Source: CAD feature listing. Evaluate the final solid. Frame: model axes, mm. A direction names the side the tool comes from. Round coordinates to 2 decimals unless told otherwise and drop trailing zeros. Order: outer loops, then holes, each group sorted by start corner. A loop starts at its lowest first (then second) coordinate and runs counter-clockwise, first axis right, second up. Notation, with made-up numbers: (84, 81.5) - (113, 81.5) arc R20 cw to (113, 90.5) - close; hole circle Ø7 at (79, 19.5). An arc over 180 degrees is marked (long way). Put each result on its own line as item: value. Start each with the question number.
1) Line query: probe 1 along X at (y, z) = (-3.5, 1.75); probe 2 along Y at (x, z) = (-6.5, -1); probe 3 along Y at (x, z) = (0.75, 2.25). Output: solid intervals per line, ascending. Write a range as [from, to].
2) Mould query, pull axis X, two halves, no side actions, for faces 1 (the face through (-6, -3.25, 2)), 2 (the face through (7, -5, -1)), 3 (the face through (-6.24, 3.826, -3.073)). Classes: +X half, -X half, draft (parallel to the pull), parting line (faces both ways), or undercut.
3) Section C-C on x = 3.25. Output: boundary loops of the cut face in (y, z), then the cut area to 3 significant figures.
4) Access query for faces 4 (the face through (-5, 2, 2)), 5 (the face through (-6.6, -5.75, -1.5)), 6 (the face through (-4, 0, 4.2)), 7 (the face through (-6.6, 3.75, -1.5)), 8 (the face through (0, 5, 1)). Directions: +Z, -Z, +X, -X, +Y, -Y. A direction counts if a zero-diameter tool reaches every point of the face in a straight line with its end or side. Return the directions, or none.
5) Section D-D on y = 3.5. Output: boundary loops of the cut face in (x, z) (3 decimals), then the cut area to 3 significant figures.
6) Section A-A on y = -3. Output: boundary loops of the cut face in (x, z).
7) Contact query for flat-ended pins moving along their axis: P1, Ø1.5, axis at y = 5, z = 3, coming from the +X side; P2, Ø1.2, axis at y = -0.5, z = 1.5, coming from the +X side (3 decimals); P3, Ø2, axis at y = -5.5, z = -0.5, coming from the +X side; P4, Ø0.6, axis at x = 6, y = 5, coming from the +Z side. Output: stop coordinate, or through.
8) Section B-B on z = -1. Output: boundary loops of the cut face in (x, y), then the cut area to 3 significant figures.
```python
from build123d import *
from OCP.BRepFilletAPI import BRepFilletAPI_MakeChamfer

# Parameters (mm, degrees)
ESQUISSE1_W             = 14.5
ESQUISSE1_H             = 14.5
BOSS_EXTRU_1_DEPTH      = 5
ESQUISSE2_W             = 8
ESQUISSE2_H             = 6.5
ENL_V_MAT_EXTRU_1_DEPTH = 12.407234547
CHANFREIN1_SIZE         = 5
CHANFREIN1_SIZE_2       = 1.75
CHANFREIN2_SIZE         = 5
CHANFREIN2_SIZE_2       = 3
ESQUISSE3_W             = 2
ESQUISSE3_H             = 4
ENL_V_MAT_EXTRU_2_DEPTH = 3.5
ESQUISSE6_W             = 10
ESQUISSE6_H             = 3
ENL_V_MAT_EXTRU_3_DEPTH = 4
CHANFREIN3_SIZE         = 4
CHANFREIN3_SIZE2        = 1.5
CONG_1_R                = 2
ESQUISSE7_W             = 1.25
ESQUISSE7_H             = 4
ENL_V_MAT_EXTRU_4_DEPTH = 4
ESQUISSE8_W             = 1.5
ESQUISSE8_H             = 2
BOSS_EXTRU_2_DEPTH      = 4
CHANFREIN4_SIZE         = 0.2
CHANFREIN4_SIZE2        = 1.5
CHANFREIN5_SIZE         = 1.5
CHANFREIN5_SIZE2        = 0.2
CHANFREIN6_SIZE         = 0.5
CHANFREIN6_SIZE2        = 1.5
CHANFREIN7_SIZE         = 1.5
CHANFREIN7_SIZE2        = 0.5
ESQUISSE9_W             = 1
ESQUISSE9_H             = 3
ENL_V_MAT_EXTRU_5_DEPTH = 3.5
ESQUISSE10_W            = 4.75
ESQUISSE10_H            = 1
ENL_V_MAT_EXTRU_6_DEPTH = 12.407234547
ESQUISSE11_W            = 1.5
ESQUISSE11_H            = 0.5
ENL_V_MAT_EXTRU_7_DEPTH = 4.25
CONG_2_START            = -3.497851783
CONG_2_DEPTH            = 7


with BuildPart() as part:
    # Esquisse1 → Boss.-Extru.1 (new body)
    with BuildSketch(Plane.XY):
        Rectangle(ESQUISSE1_W, ESQUISSE1_H)
    extrude(amount=BOSS_EXTRU_1_DEPTH)

    # Esquisse2 → Enlèv. mat.-Extru.1 (cut, through all)
    with BuildSketch(Plane.XY.offset(5)):
        Rectangle(ESQUISSE2_W, ESQUISSE2_H)
    extrude(amount=-ENL_V_MAT_EXTRU_1_DEPTH, mode=Mode.SUBTRACT)

    # Chanfrein1
    # the kernel refuses this chamfer: 5, 1.75 mm, written as the material it takes off along each edge
    with BuildSketch(Plane(origin=(7.25, 20.222980747, 5), x_dir=(0, 0, -1), z_dir=(0, -1, 0)), Plane(origin=(-7.25, -20.222980747, 5), x_dir=(0, 0, -1), z_dir=(0, 1, 0))) as chanfrein1_piece_1:
        Polygon((CHANFREIN1_SIZE, 0), (0, -CHANFREIN1_SIZE_2), (0, 0), align=None)
    extrude(amount=40.445961493, mode=Mode.SUBTRACT)

    # Chanfrein2
    # the kernel refuses this chamfer: 5, 3 mm, written as the material it takes off along each edge
    with BuildSketch(Plane(origin=(-18.431305486, 7.25, 5), x_dir=(0, 0, -1), z_dir=(1, 0, 0))) as chanfrein2_piece_1:
        Polygon((CHANFREIN2_SIZE, 0), (0, -CHANFREIN2_SIZE_2), (0, 0), align=None)
    extrude(amount=36.862610972, mode=Mode.SUBTRACT)

    # Esquisse3 → Enlèv. mat.-Extru.2 (cut)
    with BuildSketch(Plane.XY.offset(5)):
        with Locations((-6.25, 5.25)):
            Rectangle(ESQUISSE3_W, ESQUISSE3_H)
        with Locations((6.25, 5.25)):
            Rectangle(ESQUISSE3_W, ESQUISSE3_H)
        with Locations((6.25, -5.25)):
            Rectangle(ESQUISSE3_W, ESQUISSE3_H)
        with Locations((-6.25, -5.25)):
            Rectangle(ESQUISSE3_W, ESQUISSE3_H)
    extrude(amount=-ENL_V_MAT_EXTRU_2_DEPTH, mode=Mode.SUBTRACT)

    # Esquisse6 → Enlèv. mat.-Extru.3 (cut)
    with BuildSketch(Plane.XY.offset(5)):
        with Locations((0, 5.75)):
            Rectangle(ESQUISSE6_W, ESQUISSE6_H)
    extrude(amount=-ENL_V_MAT_EXTRU_3_DEPTH, mode=Mode.SUBTRACT)

    # Chanfrein3
    chanfrein3_edges = [part.edges().sort_by_distance(p)[0] for p in [
        (0, -7.25, 5),
    ]]
    chanfrein3_side = [part.faces().sort_by_distance(p)[0] for p in [
        (0, -7.25, 2.338531514),
    ]]
    chamfer(chanfrein3_edges, length=CHANFREIN3_SIZE, length2=CHANFREIN3_SIZE2, reference=chanfrein3_side[0])

    # Congé1
    cong_1_edges = [part.edges().sort_by_distance(p)[0] for p in [
        (0, -5.75, 5),
    ]]
    fillet(cong_1_edges, radius=CONG_1_R)

    # Esquisse7 → Enlèv. mat.-Extru.4 (cut)
    with BuildSketch(Plane(origin=(0, 0, 0), x_dir=(-1, 0, 0), z_dir=(0, 0, -1))):
        with Locations((-4.625, 0)):
            Rectangle(ESQUISSE7_W, ESQUISSE7_H)
        with Locations((4.625, 0)):
            Rectangle(ESQUISSE7_W, ESQUISSE7_H)
    extrude(amount=-ENL_V_MAT_EXTRU_4_DEPTH, mode=Mode.SUBTRACT)

    # Esquisse8 → Boss.-Extru.2 (add)
    with BuildSketch(Plane(origin=(0, 0, 0), x_dir=(-1, 0, 0), z_dir=(0, 0, -1))):
        with Locations((-6.25, 4.75)):
            Rectangle(ESQUISSE8_W, ESQUISSE8_H)
        with Locations((6.25, 4.75)):
            Rectangle(ESQUISSE8_W, ESQUISSE8_H)
        with Locations((6.25, -4.75)):
            Rectangle(ESQUISSE8_W, ESQUISSE8_H)
        with Locations((-6.25, -4.75)):
            Rectangle(ESQUISSE8_W, ESQUISSE8_H)
    extrude(amount=BOSS_EXTRU_2_DEPTH)

    # Chanfrein4: one chamfer whose edges measure the first distance from different faces: ONE call of the kernel's chamfer builder (chamfer() names one face for all edges)
    chanfrein4_edges_1 = [part.edges().sort_by_distance(p)[0] for p in [
        (6.25, 5.75, -4),
    ]]
    chanfrein4_side_1 = [part.faces().sort_by_distance(p)[0] for p in [
        (6.25, 4.75, -4),
    ]]
    chanfrein4_edges_2 = [part.edges().sort_by_distance(p)[0] for p in [
        (-6.25, 3.75, -4),
        (-6.25, 5.75, -4),
    ]]
    chanfrein4_side_2 = [part.faces().sort_by_distance(p)[0] for p in [
        (-6.25, 4.75, -4),
    ]]
    chanfrein4_edges_3 = [part.edges().sort_by_distance(p)[0] for p in [
        (6.25, -3.75, -4),
    ]]
    chanfrein4_side_3 = [part.faces().sort_by_distance(p)[0] for p in [
        (6.25, -4.75, -4),
    ]]
    chanfrein4 = BRepFilletAPI_MakeChamfer(part.part.solid().wrapped)
    for e in chanfrein4_edges_1:
        chanfrein4.Add(CHANFREIN4_SIZE, CHANFREIN4_SIZE2, e.wrapped, chanfrein4_side_1[0].wrapped)  # the first distance lies on this face
    for e in chanfrein4_edges_2:
        chanfrein4.Add(CHANFREIN4_SIZE, CHANFREIN4_SIZE2, e.wrapped, chanfrein4_side_2[0].wrapped)  # the first distance lies on this face
    for e in chanfrein4_edges_3:
        chanfrein4.Add(CHANFREIN4_SIZE, CHANFREIN4_SIZE2, e.wrapped, chanfrein4_side_3[0].wrapped)  # the first distance lies on this face
    add(Compound.cast(chanfrein4.Shape()), mode=Mode.REPLACE)

    # Chanfrein5: one chamfer whose edges measure the first distance from different faces: ONE call of the kernel's chamfer builder (chamfer() names one face for all edges)
    chanfrein5_edges_1 = [part.edges().sort_by_distance(p)[0] for p in [
        (6.25, 3.75, -4),
    ]]
    chanfrein5_side_1 = [part.faces().sort_by_distance(p)[0] for p in [
        (6.25, 3.75, -2),
    ]]
    chanfrein5_edges_2 = [part.edges().sort_by_distance(p)[0] for p in [
        (-6.25, -5.75, -4),
    ]]
    chanfrein5_side_2 = [part.faces().sort_by_distance(p)[0] for p in [
        (-6.25, -5.75, -2),
    ]]
    chanfrein5_edges_3 = [part.edges().sort_by_distance(p)[0] for p in [
        (-6.25, -3.75, -4),
    ]]
    chanfrein5_side_3 = [part.faces().sort_by_distance(p)[0] for p in [
        (-6.25, -3.75, -2),
    ]]
    chanfrein5_edges_4 = [part.edges().sort_by_distance(p)[0] for p in [
        (6.25, -5.75, -4),
    ]]
    chanfrein5_side_4 = [part.faces().sort_by_distance(p)[0] for p in [
        (6.25, -5.75, -2),
    ]]
    chanfrein5 = BRepFilletAPI_MakeChamfer(part.part.solid().wrapped)
    for e in chanfrein5_edges_1:
        chanfrein5.Add(CHANFREIN5_SIZE, CHANFREIN5_SIZE2, e.wrapped, chanfrein5_side_1[0].wrapped)  # the first distance lies on this face
    for e in chanfrein5_edges_2:
        chanfrein5.Add(CHANFREIN5_SIZE, CHANFREIN5_SIZE2, e.wrapped, chanfrein5_side_2[0].wrapped)  # the first distance lies on this face
    for e in chanfrein5_edges_3:
        chanfrein5.Add(CHANFREIN5_SIZE, CHANFREIN5_SIZE2, e.wrapped, chanfrein5_side_3[0].wrapped)  # the first distance lies on this face
    for e in chanfrein5_edges_4:
        chanfrein5.Add(CHANFREIN5_SIZE, CHANFREIN5_SIZE2, e.wrapped, chanfrein5_side_4[0].wrapped)  # the first distance lies on this face
    add(Compound.cast(chanfrein5.Shape()), mode=Mode.REPLACE)

    # Chanfrein6: one chamfer whose edges measure the first distance from different faces: ONE call of the kernel's chamfer builder (chamfer() names one face for all edges)
    chanfrein6_edges_1 = [part.edges().sort_by_distance(p)[0] for p in [
        (5.5, 4.75, -4),
    ]]
    chanfrein6_side_1 = [part.faces().sort_by_distance(p)[0] for p in [
        (6.25, 4.75, -4),
    ]]
    chanfrein6_edges_2 = [part.edges().sort_by_distance(p)[0] for p in [
        (-7, 4.75, -4),
    ]]
    chanfrein6_side_2 = [part.faces().sort_by_distance(p)[0] for p in [
        (-6.25, 4.75, -4),
    ]]
    chanfrein6_edges_3 = [part.edges().sort_by_distance(p)[0] for p in [
        (-5.5, -4.75, -4),
        (-7, -4.75, -4),
    ]]
    chanfrein6_side_3 = [part.faces().sort_by_distance(p)[0] for p in [
        (-6.25, -4.75, -4),
    ]]
    chanfrein6 = BRepFilletAPI_MakeChamfer(part.part.solid().wrapped)
    for e in chanfrein6_edges_1:
        chanfrein6.Add(CHANFREIN6_SIZE, CHANFREIN6_SIZE2, e.wrapped, chanfrein6_side_1[0].wrapped)  # the first distance lies on this face
    for e in chanfrein6_edges_2:
        chanfrein6.Add(CHANFREIN6_SIZE, CHANFREIN6_SIZE2, e.wrapped, chanfrein6_side_2[0].wrapped)  # the first distance lies on this face
    for e in chanfrein6_edges_3:
        chanfrein6.Add(CHANFREIN6_SIZE, CHANFREIN6_SIZE2, e.wrapped, chanfrein6_side_3[0].wrapped)  # the first distance lies on this face
    add(Compound.cast(chanfrein6.Shape()), mode=Mode.REPLACE)

    # Chanfrein7: one chamfer whose edges measure the first distance from different faces: ONE call of the kernel's chamfer builder (chamfer() names one face for all edges)
    chanfrein7_edges_1 = [part.edges().sort_by_distance(p)[0] for p in [
        (5.5, -4.75, -4),
    ]]
    chanfrein7_side_1 = [part.faces().sort_by_distance(p)[0] for p in [
        (5.5, -4.75, -1.941558442),
    ]]
    chanfrein7_edges_2 = [part.edges().sort_by_distance(p)[0] for p in [
        (-5.5, 4.75, -4),
    ]]
    chanfrein7_side_2 = [part.faces().sort_by_distance(p)[0] for p in [
        (-5.5, 4.75, -1.941558442),
    ]]
    chanfrein7_edges_3 = [part.edges().sort_by_distance(p)[0] for p in [
        (7, 4.75, -4),
    ]]
    chanfrein7_side_3 = [part.faces().sort_by_distance(p)[0] for p in [
        (7, 4.75, -1.941558442),
    ]]
    chanfrein7_edges_4 = [part.edges().sort_by_distance(p)[0] for p in [
        (7, -4.75, -4),
    ]]
    chanfrein7_side_4 = [part.faces().sort_by_distance(p)[0] for p in [
        (7, -4.75, -1.941558442),
    ]]
    chanfrein7 = BRepFilletAPI_MakeChamfer(part.part.solid().wrapped)
    for e in chanfrein7_edges_1:
        chanfrein7.Add(CHANFREIN7_SIZE, CHANFREIN7_SIZE2, e.wrapped, chanfrein7_side_1[0].wrapped)  # the first distance lies on this face
    for e in chanfrein7_edges_2:
        chanfrein7.Add(CHANFREIN7_SIZE, CHANFREIN7_SIZE2, e.wrapped, chanfrein7_side_2[0].wrapped)  # the first distance lies on this face
    for e in chanfrein7_edges_3:
        chanfrein7.Add(CHANFREIN7_SIZE, CHANFREIN7_SIZE2, e.wrapped, chanfrein7_side_3[0].wrapped)  # the first distance lies on this face
    for e in chanfrein7_edges_4:
        chanfrein7.Add(CHANFREIN7_SIZE, CHANFREIN7_SIZE2, e.wrapped, chanfrein7_side_4[0].wrapped)  # the first distance lies on this face
    add(Compound.cast(chanfrein7.Shape()), mode=Mode.REPLACE)

    # Esquisse9 → Enlèv. mat.-Extru.5 (cut)
    with BuildSketch(Plane.XY.offset(1.5)):
        with Locations((-5.75, 4.75)):
            Rectangle(ESQUISSE9_W, ESQUISSE9_H)
        with Locations((-5.75, -4.75)):
            Rectangle(ESQUISSE9_W, ESQUISSE9_H)
        with Locations((5.75, -4.75)):
            Rectangle(ESQUISSE9_W, ESQUISSE9_H)
        with Locations((5.75, 4.75)):
            Rectangle(ESQUISSE9_W, ESQUISSE9_H)
    extrude(amount=-ENL_V_MAT_EXTRU_5_DEPTH, mode=Mode.SUBTRACT)

    # Esquisse10 → Enlèv. mat.-Extru.6 (cut, through all)
    with BuildSketch(Plane.XY.offset(1)):
        with Locations((-2.625, 5.5)):
            Rectangle(ESQUISSE10_W, ESQUISSE10_H)
        with Locations((2.625, 5.5)):
            Rectangle(ESQUISSE10_W, ESQUISSE10_H)
    extrude(amount=-ENL_V_MAT_EXTRU_6_DEPTH, mode=Mode.SUBTRACT)

    # Esquisse11 → Enlèv. mat.-Extru.7 (cut)
    with BuildSketch(Plane(origin=(0, 0, 0), x_dir=(-1, 0, 0), z_dir=(0, 0, -1))):
        Polygon((-3.502148217, -3.75), (-3.502148217, -5.75), (0, -5.75), (3.497851783, -5.75), (3.497851783, -3.75), align=None)
        with Locations((2.747851783, -3.5)):
            Rectangle(ESQUISSE11_W, ESQUISSE11_H)
        with Locations((-2.752148217, -3.5)):
            Rectangle(ESQUISSE11_W, ESQUISSE11_H)
    extrude(amount=-ENL_V_MAT_EXTRU_7_DEPTH, mode=Mode.SUBTRACT)

    # Congé2: read off the stored shape, not the designer's step
    # Congé2 outline → Congé2 (add)
    with BuildSketch(Plane.YZ.offset(CONG_2_START)):
        with BuildLine():
            Line((-5.75, 4.25), (-5.75, 2.25))
            ThreePointArc((-5.75, 2.25), (-5.164213562, 3.664213562), (-3.75, 4.25))
            Line((-3.75, 4.25), (-5.75, 4.25))
        make_face()
    extrude(amount=CONG_2_DEPTH)


solid = part.part
```
Answer sheet:
1. probe 1: [-5.25, -3.5], [-2, 2], [3.5, 5.25]
1. probe 2: [-5.75, -3.75], [3.75, 5.75]
1. probe 3: [-6.78, -5.75], [-3.75, -3.25], [3.25, 4.25]
2. face 1: undercut
2. face 2: +X half
2. face 3: draft
3. outline: (-7.25, 0) - (-5.75, 0) - (-5.75, 2.25) arc R2 cw to (-3.75, 4.25) - (-3.25, 4.25) - (-3.25, 5) - (-4.36, 5) arc R2 ccw to (-6.24, 3.7) - (-7.25, 1) - close; (3.25, 0) - (5, 0) - (5, 1) - (4.25, 1) - (4.25, 5) - (3.25, 5) - close; (6, 0) - (7.25, 0) - (6.65, 1) - (6, 1) - close
3. area: 13.6 mm^2
4. face 4: -Z
4. face 5: -Z, +X, -X, -Y
4. face 6: +Z, -Z
4. face 7: -Z, +X, -X
4. face 8: +Z, +Y
5. outline: (-7.25, 0) - (-6.25, 0) - (-6.25, 1.5) - (-6.725, 1.5) - close; (-5.25, 0) - (5.25, 0) - (5.25, 5) - (-5.25, 5) - close; (6.25, 0) - (7.25, 0) - (6.725, 1.5) - (6.25, 1.5) - close
5. area: 54.7 mm^2
6. outline: (-7.25, 0) - (-4, 0) - (-4, 5) - (-5.5, 5) - close; (4, 0) - (7.25, 0) - (5.5, 5) - (4, 5) - close
7. P1: x = 5.25
7. P2: x = 6.935
7. P3: x = 7.25
7. P4: z = 1.5
8. outline: (-7, -5.75) - (-6.25, -5.75) - (-6.25, -3.75) - (-7, -3.75) - close; (-7, 3.75) - (-6.25, 3.75) - (-6.25, 5.75) - (-7, 5.75) - close; (6.25, -5.75) - (7, -5.75) - (7, -3.75) - (6.25, -3.75) - close; (6.25, 3.75) - (7, 3.75) - (7, 5.75) - (6.25, 5.75) - close
8. area: 6.00 mm^2
